```python
from build123d import *

# Parameters (mm, degrees)
F1_W           = 100.3
F1_H           = 141.77
F2_DEPTH       = 60
F3_T           = -3
F4_R           = 2
F5_DEPTH       = 25
F6_W           = 80
F6_H           = 30
F7_DEPTH       = 25
F8_W           = 105.77
F8_H           = 18.364803344
F9_DEPTH       = 25
F10_W          = 70.3
F10_H          = 10
F11_DEPTH      = 25
F12_R          = 2.25
F13_DEPTH      = 25
F15_DEPTH      = 8
F17_DEPTH      = 8
F19_R          = 1.25
F18_R          = 1.25
F20_R          = 1.25
F21_R          = 1.25
F22_DEPTH      = 25
F23_R          = 5
F24_R          = 5
F25_R          = 3
F26_DEPTH      = 25
F27_W          = 7
F27_H          = 40
F28_DEPTH      = 25
F29_R          = 3.49999
F31_DEPTH      = 25
F32_R          = 2.5
F32_R_2        = 1
F33_DEPTH      = 3
F33_DEPTH_BACK = 3


# Not quite as in the source:
# - a fillet or chamfer is up to 0.001 mm smaller than in the source, because OpenCascade refuses the exact size


with BuildPart() as f2:
    # F1 (on face) → F2 (new body)
    with BuildSketch(Plane.XY):
        with Locations((-6.5499655962, -8.0085539126)):
            Rectangle(F1_W, F1_H)
    extrude(amount=F2_DEPTH)

    # F3
    f3_openings = [f2.faces().sort_by_distance(p)[0] for p in [
        (-6.549966, -8.008554, 60),
    ]]
    offset(amount=F3_T, openings=f3_openings)

    # F4 (on face) → F5 (cut)
    with BuildSketch(Plane.XY.offset(3)):
        with Locations((-34.1999655962, 31.3764460874)):
            Circle(F4_R)
        with Locations((14.6000344038, 37.7764460874)):
            Circle(F4_R)
        with Locations((14.5000344038, -44.6235539126)):
            Circle(F4_R)
        with Locations((-34.1999655962, -43.3235539126)):
            Circle(F4_R)
    extrude(amount=-F5_DEPTH, mode=Mode.SUBTRACT)

    # F6 (on face) → F7 (cut)
    with BuildSketch(Plane.XZ.offset(78.8935539126)):
        with Locations((-6.6999655962, 20)):
            Rectangle(F6_W, F6_H)
    extrude(amount=-F7_DEPTH, mode=Mode.SUBTRACT)

    # F8 (on face) → F9 (cut)
    with BuildSketch(Plane.YZ.offset(43.6000344038)):
        with Locations((-8.0085539126, 50.817598328)):
            Rectangle(F8_W, F8_H)
    extrude(amount=-F9_DEPTH, mode=Mode.SUBTRACT)

    # F10 (on face) → F11 (cut)
    with BuildSketch(Plane(origin=(0, 62.8764460874, 0), x_dir=(-1, 0, 0), z_dir=(0, 1, 0))):
        with Locations((6.5499655962, 55)):
            Rectangle(F10_W, F10_H)
    extrude(amount=-F11_DEPTH, mode=Mode.SUBTRACT)

    # F12 (on face) → F13 (cut)
    with BuildSketch(Plane.XY.offset(3)):
        with Locations((-46.6999655962, 52.8764460874)):
            Circle(F12_R)
        with Locations((33.6000344038, 52.8764460874)):
            Circle(F12_R)
        with Locations((-46.6999655962, -68.8935539126)):
            Circle(F12_R)
    extrude(amount=-F13_DEPTH, mode=Mode.SUBTRACT)

    # F14 (on face) → F15 (join)
    with BuildSketch(Plane.YZ.offset(-53.6999655962)):
        Polygon((59.8764460874, 44), (59.8764460874, 57), (51.8764460874, 57), (51.8764460874, 52), align=None)
        Polygon((-75.8935539126, 57), (-75.8935539126, 44), (-67.8935539126, 52), (-67.8935539126, 57), align=None)
    extrude(amount=F15_DEPTH)

    # F16 (on face) → F17 (join)
    with BuildSketch(Plane(origin=(40.6000344038, 0, 0), x_dir=(0, -1, 0), z_dir=(-1, 0, 0))):
        Polygon((-59.8764460874, 57), (-59.8764460874, 44), (-51.8764460874, 52), (-51.8764460874, 57), align=None)
        Polygon((75.8935539126, 57), (67.8935539126, 57), (67.8935539126, 52), (75.8935539126, 44), align=None)
    extrude(amount=F17_DEPTH)

    # F19 (on face) + F18 (on face) + F20 (on face) + F21 (on face) → F22 (cut)
    with BuildSketch(Plane.XY.offset(57)):
        with Locations((-49.6999655962, 55.8764460874)):
            Circle(F19_R)
    with BuildSketch(Plane.XY.offset(57)):
        with Locations((36.6000344038, 55.8764460874)):
            Circle(F18_R)
    with BuildSketch(Plane.XY.offset(57)):
        with Locations((-49.6999655962, -71.8935539126)):
            Circle(F20_R)
    with BuildSketch(Plane.XY.offset(57)):
        with Locations((36.6000344038, -71.8935539126)):
            Circle(F21_R)
    extrude(amount=-F22_DEPTH, mode=Mode.SUBTRACT)

    # F23
    f23_edges = [f2.edges().sort_by_distance(p)[0] for p in [
        (-45.699966, 51.876446, 54.5),
        (32.600034, 51.876446, 54.5),
        (-45.699966, -67.893554, 54.5),
        (32.600034, -67.893554, 54.5),
    ]]
    fillet(f23_edges, radius=F23_R)

    # F24
    f24_edges = [f2.edges().sort_by_distance(p)[0] for p in [
        (43.600034, 62.876446, 30),
        (-56.699966, 62.876446, 30),
        (-56.699966, -78.893554, 30),
        (43.600034, -78.893554, 30),
    ]]
    fillet(f24_edges, radius=F24_R)

    # F25 (on face) → F26 (cut)
    with BuildSketch(Plane.YZ.offset(43.6000344038)):
        with Locations((-3.5735539126, 22.5)):
            Circle(F25_R)
    extrude(amount=-F26_DEPTH, mode=Mode.SUBTRACT)

    # F27 (on face) → F28 (cut)
    with BuildSketch(Plane(origin=(-56.6999655962, 0, 0), x_dir=(0, -1, 0), z_dir=(-1, 0, 0))):
        with Locations((-43.8384013922, 28.5368594155)):
            Rectangle(F27_W, F27_H)
    extrude(amount=-F28_DEPTH, mode=Mode.SUBTRACT)

    # F29 (radius 3.5 in the source; OpenCascade refuses exactly that, so slightly less here)
    f29_edges = [f2.edges().sort_by_distance(p)[0] for p in [
        (-55.199966, 40.338401, 48.536859),
        (-55.199966, 47.338401, 48.536859),
        (-55.199966, 40.338401, 8.536859),
        (-55.199966, 47.338401, 8.536859),
    ]]
    fillet(f29_edges, radius=F29_R)

    # F30 (on face) → F31 (cut)
    with BuildSketch(Plane(origin=(-56.6999655962, 0, 0), x_dir=(0, -1, 0), z_dir=(-1, 0, 0))):
        with BuildLine():
            Line((-40.3384013922, 12.0368594155), (-40.3384013922, 45.0368594155))
            ThreePointArc((-40.3384013922, 45.0368594155), (-43.8384013922, 48.5368594155), (-47.3384013922, 45.0368594155))
            Line((-47.3384013922, 45.0368594155), (-47.3384013922, 12.0368594155))
            ThreePointArc((-47.3384013922, 12.0368594155), (-43.8384013922, 8.5368594155), (-40.3384013922, 12.0368594155))
        make_face()
        with BuildLine():
            Line((-28.8384013922, 12.0368594155), (-28.8384013922, 45.0368594155))
            ThreePointArc((-28.8384013922, 45.0368594155), (-32.3384013922, 48.5368594155), (-35.8384013922, 45.0368594155))
            Line((-35.8384013922, 45.0368594155), (-35.8384013922, 12.0368594155))
            ThreePointArc((-35.8384013922, 12.0368594155), (-32.3384013922, 8.5368594155), (-28.8384013922, 12.0368594155))
        make_face()
        with BuildLine():
            Line((-17.3384013922, 12.0368594155), (-17.3384013922, 45.0368594155))
            ThreePointArc((-17.3384013922, 45.0368594155), (-20.8384013922, 48.5368594155), (-24.3384013922, 45.0368594155))
            Line((-24.3384013922, 45.0368594155), (-24.3384013922, 12.0368594155))
            ThreePointArc((-24.3384013922, 12.0368594155), (-20.8384013922, 8.5368594155), (-17.3384013922, 12.0368594155))
        make_face()
        with BuildLine():
            Line((-5.8384013922, 12.0368594155), (-5.8384013922, 45.0368594155))
            ThreePointArc((-5.8384013922, 45.0368594155), (-9.3384013922, 48.5368594155), (-12.8384013922, 45.0368594155))
            Line((-12.8384013922, 45.0368594155), (-12.8384013922, 12.0368594155))
            ThreePointArc((-12.8384013922, 12.0368594155), (-9.3384013922, 8.5368594155), (-5.8384013922, 12.0368594155))
        make_face()
        with BuildLine():
            Line((5.6615986078, 12.0368594155), (5.6615986078, 45.0368594155))
            ThreePointArc((5.6615986078, 45.0368594155), (2.1615986078, 48.5368594155), (-1.3384013922, 45.0368594155))
            Line((-1.3384013922, 45.0368594155), (-1.3384013922, 12.0368594155))
            ThreePointArc((-1.3384013922, 12.0368594155), (2.1615986078, 8.5368594155), (5.6615986078, 12.0368594155))
        make_face()
        with BuildLine():
            Line((17.1615986078, 12.0368594155), (17.1615986078, 45.0368594155))
            ThreePointArc((17.1615986078, 45.0368594155), (13.6615986078, 48.5368594155), (10.1615986078, 45.0368594155))
            Line((10.1615986078, 45.0368594155), (10.1615986078, 12.0368594155))
            ThreePointArc((10.1615986078, 12.0368594155), (13.6615986078, 8.5368594155), (17.1615986078, 12.0368594155))
        make_face()
        with BuildLine():
            Line((28.6615986078, 12.0368594155), (28.6615986078, 45.0368594155))
            ThreePointArc((28.6615986078, 45.0368594155), (25.1615986078, 48.5368594155), (21.6615986078, 45.0368594155))
            Line((21.6615986078, 45.0368594155), (21.6615986078, 12.0368594155))
            ThreePointArc((21.6615986078, 12.0368594155), (25.1615986078, 8.5368594155), (28.6615986078, 12.0368594155))
        make_face()
        with BuildLine():
            Line((40.1615986078, 12.0368594155), (40.1615986078, 45.0368594155))
            ThreePointArc((40.1615986078, 45.0368594155), (36.6615986078, 48.5368594155), (33.1615986078, 45.0368594155))
            Line((33.1615986078, 45.0368594155), (33.1615986078, 12.0368594155))
            ThreePointArc((33.1615986078, 12.0368594155), (36.6615986078, 8.5368594155), (40.1615986078, 12.0368594155))
        make_face()
        with BuildLine():
            Line((51.6615986078, 12.0368594155), (51.6615986078, 45.0368594155))
            ThreePointArc((51.6615986078, 45.0368594155), (48.1615986078, 48.5368594155), (44.6615986078, 45.0368594155))
            Line((44.6615986078, 45.0368594155), (44.6615986078, 12.0368594155))
            ThreePointArc((44.6615986078, 12.0368594155), (48.1615986078, 8.5368594155), (51.6615986078, 12.0368594155))
        make_face()
        with BuildLine():
            Line((63.1615986078, 12.0368594155), (63.1615986078, 45.0368594155))
            ThreePointArc((63.1615986078, 45.0368594155), (59.6615986078, 48.5368594155), (56.1615986078, 45.0368594155))
            Line((56.1615986078, 45.0368594155), (56.1615986078, 12.0368594155))
            ThreePointArc((56.1615986078, 12.0368594155), (59.6615986078, 8.5368594155), (63.1615986078, 12.0368594155))
        make_face()
    extrude(amount=-F31_DEPTH, mode=Mode.SUBTRACT)

    # F32 (on face) → F33 (join, two sides)
    with BuildSketch(Plane.XY.offset(3)) as f33_sk:
        with Locations((14.6000344038, 37.7764460874)):
            Circle(F32_R)
        with Locations((14.6000344038, 37.7764460874)):
            Circle(F32_R_2, mode=Mode.SUBTRACT)
        with Locations((14.5000344038, -44.6235539126)):
            Circle(F32_R)
        with Locations((14.5000344038, -44.6235539126)):
            Circle(F32_R_2, mode=Mode.SUBTRACT)
        with Locations((-34.1999655962, -43.3235539126)):
            Circle(F32_R)
        with Locations((-34.1999655962, -43.3235539126)):
            Circle(F32_R_2, mode=Mode.SUBTRACT)
        with Locations((-34.1999655962, 31.3764460874)):
            Circle(F32_R)
        with Locations((-34.1999655962, 31.3764460874)):
            Circle(F32_R_2, mode=Mode.SUBTRACT)
    extrude(amount=F33_DEPTH)
    extrude(f33_sk.sketch, amount=-F33_DEPTH_BACK)


solid = f2.part
```
Geometry: final body of the model. Coordinates: model frame, mm. A direction names the side the tool comes from. Coordinates: 2 decimals unless noted, no trailing zeros. Write each loop counter-clockwise with the first axis right and the second up, starting at its lowest first coordinate (ties: lowest second). Pieces come first, ordered by that corner, then holes. Notation, with made-up numbers: M -22.5,30 L -1.5,30 A26 cw -1.5,64 Z; hole C 36,-3.5 d10. An arc over 180 degrees is marked long. Use CSV: the item, a comma, the result in double quotes. Start each with the question number.
1. Ray query, probe 1 along Y at (x, z) = (-49, 21); probe 2 along X at (y, z) = (-62.5, 4); probe 3 along X at (y, z) = (-10, 49). Return the intervals inside material, ascending.
2. Cut plane C-C on z = 37. Count the separate pieces of the cut face and the enclosed holes in it, plus the area to 3 significant figures.
3. First-contact query: P1, Ø1.2, axis at x = -34.2, y = 31.38, coming from the +Z side; P2, Ø3, axis at x = 36.6, y = 55.88, coming from the +Z side; P3, Ø8, axis at y = -55.5, z = 48.5, coming from the +X side; P4, Ø1.5, axis at x = -55, z = 35, coming from the +Y side. Flat tips, straight axial feed; report the tip coordinate or a pass-through.
4. Reachability of faces 1 (the face through (-55.221, 9.261, 48.536)), 2 (the face through (38.434, 55.932, 47.944)), 3 (the face through (-55.221, -59.585, 8.538)) from +Z, -Z, +X, -X, +Y, -Y: full face, straight path, thin tool, end or side. Return the list, or none.
5. Mould query, pull axis Z, two halves, no side actions, for faces 4 (the face through (-55.221, -59.739, 48.536)), 5 (the face through (42, -60.894, 51)), 6 (the face through (41, 56, 60)). Classes: pulls with the +Z half, pulls with the -Z half, needs draft (parallel to the pull), parting line crosses it, or undercut.
6. Cut plane B-B on y = -3.5. Return the cut outline in (x, z).
7. Cut plane A-A on x = -18. Return the cut outline in (y, z), plus the area to 3 significant figures.
Entries:
1,probe 1,"-78.89 to -75.89, 59.88 to 62.88"
1,probe 2,"-56.7 to -53.7, 40.6 to 43.6"
1,probe 3,"-56.7 to -53.7"
2,separate pieces,"10"
2,enclosed holes,"0"
2,area,"1,180 mm²"
3,P1,"through"
3,P2,"z = 57"
3,P3,"x = -53.7"
3,P4,"y = 62.18"
4,face 1,"+X, -X"
4,face 2,"none"
4,face 3,"-X"
5,face 4,"undercut"
5,face 5,"needs draft"
5,face 6,"pulls with the +Z half"
6,outline,"M -56.7,0 L 43.6,0 L 43.6,19.5 L 40.6,19.5 L 40.6,3 L -53.7,3 L -53.7,8.8 L -56.7,8.8 Z; M -56.7,48.27 L -53.7,48.27 L -53.7,60 L -56.7,60 Z; M 40.6,25.5 L 43.6,25.5 L 43.6,41.64 L 40.6,41.64 Z"
7,outline,"M -78.89,0 L 62.88,0 L 62.88,50 L 59.88,50 L 59.88,3 L -75.89,3 L -75.89,5 L -78.89,5 Z; M -78.89,35 L -75.89,35 L -75.89,60 L -78.89,60 Z"
7,area,"647 mm²"
